from build123d import *

# Parameters (mm, degrees)
SKETCH1_R           = 0.396875
BOSS_EXTRUDE1_DEPTH = 25.4
SKETCH3_R           = 2.29235
CUT_EXTRUDE1_DEPTH  = 45.3009


with BuildPart() as part:
    # Sketch1 → Boss-Extrude1 (new body)
    with BuildSketch(Plane(origin=(0, 0, 0), x_dir=(-1, 0, 0), z_dir=(0, 0, -1))):
        with BuildLine():
            ThreePointArc((-94.226399104, -28.701297083), (-93.354822314, -23.746772531), (-94.966890975, -18.98146097))
            ThreePointArc((-94.966890975, -18.98146097), (-92.421623219, -17.889980312), (-90.050475192, -16.459115183))
            ThreePointArc((-90.050475192, -16.459115183), (-87.119940237, -20.547993332), (-82.587097641, -22.729803966))
            ThreePointArc((-82.587097641, -22.729803966), (-81.710050828, -21.966437271), (-80.863625765, -21.169251948))
            ThreePointArc((-80.863625765, -21.169251948), (-82.5860804, -16.442719427), (-86.364828593, -13.121872888))
            ThreePointArc((-86.364828593, -13.121872888), (-84.706302386, -10.903989032), (-83.368260523, -8.479249468))
            ThreePointArc((-83.368260523, -8.479249468), (-78.785903731, -10.555054341), (-73.769441574, -10.178136478))
            ThreePointArc((-73.769441574, -10.178136478), (-73.391580101, -9.078518121), (-73.057147156, -7.964922849))
            ThreePointArc((-73.057147156, -7.964922849), (-76.912102887, -4.732852931), (-81.845018087, -3.746289563))
            ThreePointArc((-81.845018087, -3.746289563), (-81.517634186, -0.996282698), (-81.571225724, 1.772624294))
            ThreePointArc((-81.571225724, 1.772624294), (-76.564885896, 2.266102937), (-72.408961163, 5.10075446))
            ThreePointArc((-72.408961163, 5.10075446), (-72.631532707, 6.241982628), (-72.898702917, 7.373600896))
            ThreePointArc((-72.898702917, 7.373600896), (-77.853227469, 8.245177686), (-82.61853903, 6.633109025))
            ThreePointArc((-82.61853903, 6.633109025), (-83.710019688, 9.178376781), (-85.140884817, 11.549524808))
            ThreePointArc((-85.140884817, 11.549524808), (-81.052006668, 14.480059763), (-78.870196034, 19.012902359))
            ThreePointArc((-78.870196034, 19.012902359), (-79.633562729, 19.889949172), (-80.430748052, 20.736374235))
            ThreePointArc((-80.430748052, 20.736374235), (-85.157280573, 19.0139196), (-88.478127112, 15.235171407))
            ThreePointArc((-88.478127112, 15.235171407), (-90.696010968, 16.893697614), (-93.120750532, 18.231739477))
            ThreePointArc((-93.120750532, 18.231739477), (-91.044945659, 22.814096269), (-91.421863522, 27.830558426))
            ThreePointArc((-91.421863522, 27.830558426), (-92.521481879, 28.208419899), (-93.635077151, 28.542852844))
            ThreePointArc((-93.635077151, 28.542852844), (-96.867147069, 24.687897113), (-97.853710437, 19.754981913))
            ThreePointArc((-97.853710437, 19.754981913), (-100.603717302, 20.082365814), (-103.372624294, 20.028774276))
            ThreePointArc((-103.372624294, 20.028774276), (-103.866102937, 25.035114104), (-106.70075446, 29.191038837))
            ThreePointArc((-106.70075446, 29.191038837), (-107.841982628, 28.968467293), (-108.973600896, 28.701297083))
            ThreePointArc((-108.973600896, 28.701297083), (-109.845177686, 23.746772531), (-108.233109025, 18.98146097))
            ThreePointArc((-108.233109025, 18.98146097), (-110.778376781, 17.889980312), (-113.149524808, 16.459115183))
            ThreePointArc((-113.149524808, 16.459115183), (-116.080059763, 20.547993332), (-120.612902359, 22.729803966))
            ThreePointArc((-120.612902359, 22.729803966), (-121.489949172, 21.966437271), (-122.336374235, 21.169251948))
            ThreePointArc((-122.336374235, 21.169251948), (-120.6139196, 16.442719427), (-116.835171407, 13.121872888))
            ThreePointArc((-116.835171407, 13.121872888), (-118.493697614, 10.903989032), (-119.831739477, 8.479249468))
            ThreePointArc((-119.831739477, 8.479249468), (-124.414096269, 10.555054341), (-129.430558426, 10.178136478))
            ThreePointArc((-129.430558426, 10.178136478), (-129.808419899, 9.078518121), (-130.142852844, 7.964922849))
            ThreePointArc((-130.142852844, 7.964922849), (-126.287897113, 4.732852931), (-121.354981913, 3.746289563))
            ThreePointArc((-121.354981913, 3.746289563), (-121.682365814, 0.996282698), (-121.628774276, -1.772624294))
            ThreePointArc((-121.628774276, -1.772624294), (-126.635114104, -2.266102937), (-130.791038837, -5.10075446))
            ThreePointArc((-130.791038837, -5.10075446), (-130.568467293, -6.241982628), (-130.301297083, -7.373600896))
            ThreePointArc((-130.301297083, -7.373600896), (-125.346772531, -8.245177686), (-120.58146097, -6.633109025))
            ThreePointArc((-120.58146097, -6.633109025), (-119.489980312, -9.178376781), (-118.059115183, -11.549524808))
            ThreePointArc((-118.059115183, -11.549524808), (-122.147993332, -14.480059763), (-124.329803966, -19.012902359))
            ThreePointArc((-124.329803966, -19.012902359), (-123.566437271, -19.889949172), (-122.769251948, -20.736374235))
            ThreePointArc((-122.769251948, -20.736374235), (-118.042719427, -19.0139196), (-114.721872888, -15.235171407))
            ThreePointArc((-114.721872888, -15.235171407), (-112.503989032, -16.893697614), (-110.079249468, -18.231739477))
            ThreePointArc((-110.079249468, -18.231739477), (-112.155054341, -22.814096269), (-111.778136478, -27.830558426))
            ThreePointArc((-111.778136478, -27.830558426), (-110.678518121, -28.208419899), (-109.564922849, -28.542852844))
            ThreePointArc((-109.564922849, -28.542852844), (-106.332852931, -24.687897113), (-105.346289563, -19.754981913))
            ThreePointArc((-105.346289563, -19.754981913), (-102.596282698, -20.082365814), (-99.827375706, -20.028774276))
            ThreePointArc((-99.827375706, -20.028774276), (-99.333897063, -25.035114104), (-96.49924554, -29.191038837))
            ThreePointArc((-96.49924554, -29.191038837), (-95.358017372, -28.968467293), (-94.226399104, -28.701297083))
        make_face()
        with Locations((-101.6, 0)):
            Circle(SKETCH1_R, mode=Mode.SUBTRACT)
    extrude(amount=-BOSS_EXTRUDE1_DEPTH)

    # Sketch3 → Cut-Extrude1 (cut)
    with BuildSketch(Plane.XY.offset(25.4)):
        with Locations((101.6, 0)):
            Circle(SKETCH3_R)
    extrude(amount=-CUT_EXTRUDE1_DEPTH, mode=Mode.SUBTRACT)


solid = part.part
Verification items for the finished model (mm, model axes). Coordinates: 2 decimals unless noted, no trailing zeros. Loops run counter-clockwise (first coordinate to the right, second up) from the corner with the lowest first, then second, coordinate; pieces in that order, holes last. Notation, with made-up numbers: (65.25, -35) -> (103.25, -35) arc R21 cw to (103.25, -25) -> close; hole circle Ø3 at (-20, 41.25). An arc over 180 degrees is marked (long way). Answer as a JSON object with one key per item and string values. Group by question number.
Item 1: Sectioned sample at B-B on x = 101.6. Record the boundary of the cut face in (y, z), plus the area to 3 significant figures.
Item 2: Depth check by flat-ended pin: pin 1 (3.5 mm diameter, centred on x = 101.6, y = 0, fed in from -Z); pin 2 (5 mm diameter, centred on y = -12, z = 11, fed in from +X); pin 3 (5 mm diameter, centred on x = 82, z = 5, fed in from +Y); pin 4 (10 mm diameter, centred on y = 22, z = 13.5, fed in from -X). Enter the tip coordinate at first touch or a pass-through.
Item 3: Sectioned sample at C-C on y = 14.5. Record the boundary of the cut face in (x, z).
Item 4: Sectioned sample at A-A on y = 0. Record the boundary of the cut face in (x, z), plus the area to 3 significant figures.
Item 5: Mould release check, pull along Y, two halves, no side actions. Record for faces 1 (the cylindrical face through (107.83, 28.97, 12.52)), 2 (the flat face through (102, 7, 0)), 3 (the cylindrical face through (110.7, -28.2, 12.5)), 4 (the cylindrical face through (82.546, -16.502, 12.522)): +Y half, -Y half, draft (parallel to the pull), parting line (faces both ways), or undercut.
Item 6: Scan lines: probe 1 along Y at (x, z) = (101.6, 7.5); probe 2 along Y at (x, z) = (123.5, 18); probe 3 along X at (y, z) = (-17.5, 17.5). Record each from-to range of solid material in increasing order.
Evaluation:
{
 "1": {"outline": "(-20.11, 0) -> (-2.29, 0) -> (-2.29, 25.4) -> (-20.11, 25.4) -> close; (2.29, 0) -> (20.11, 0) -> (20.11, 25.4) -> (2.29, 25.4) -> close", "area": "905 mm²"},
 "2": {"pin 1": "passes through", "pin 2": "stops at x = 122.16", "pin 3": "stops at y = 20.74", "pin 4": "stops at x = 78.87"},
 "3": {"outline": "(81.04, 0) -> (118.88, 0) -> (118.88, 25.4) -> (81.04, 25.4) -> close"},
 "4": {"outline": "(81.49, 0) -> (99.31, 0) -> (99.31, 25.4) -> (81.49, 25.4) -> close; (103.89, 0) -> (121.71, 0) -> (121.71, 25.4) -> (103.89, 25.4) -> close", "area": "905 mm²"},
 "5": {"face 1": "+Y half", "face 2": "draft", "face 3": "-Y half", "face 4": "undercut"},
 "6": {"probe 1": "y = -20.11 to -2.29, 2.29 to 20.11", "probe 2": "y = -19.96 to -16.56, -7.93 to -1.66, 3.86 to 10.35", "probe 3": "x = 81.95 to 89.58, 91.7 to 111.5, 116.29 to 123.9"}
}
